Could you check a few things on this drawing? It's one solid part, dimensions in mm from its lowest x, y, z. A direction names the side the tool comes from. Give positions to 0.01 mm unless a question says otherwise; leave off trailing zeros. Order: outer loops, then holes, each group sorted by start corner. A loop starts at its lowest first (then second) coordinate and runs counter-clockwise, first axis right, second up.
(1) On a 3-axis mill with a long thin cutter (end or side, diameter ignored), from which of +Z, -Z, +X, -X, +Y, -Y can I reach the whole of each face in a straight line? I mean the marked faces 1, 2 and 3. Say none if no direction works.
(2) Imagine slicing it at A-A, the plane z = 12. State how many separate pieces and enclosed holes the cut face has.
(3) Imagine slicing it at B-B, the plane x = 14.5. Write out the boundary of the cut face in (y, z) (1 decimal).
(4) If I drill on probe 1 along Z at (x, y) = (8.5, 4.35) (1 decimal); probe 2 along X at (y, z) = (2.85, 18.5) (1 decimal); probe 3 along Z at (x, y) = (16, 4.05) (1 decimal), over which ranges is the centre line in solid material (lowest first)?
(5) Will these pins go through, and if not, where does the flat tip stop? pin 1 (1.5 mm diameter, centred on x = 18.5, y = 3.5, fed in from +Z); pin 2 (1.7 mm diameter, centred on x = 14.5, z = 5.39, fed in from -Y); pin 3 (3.5 mm diameter, centred on x = 12, z = 12, fed in from -Y); pin 4 (8 mm diameter, centred on x = 12, z = 12, fed in from +Y).
(6) If we mould it in two halves opening along Z, with no side actions, what happens to the marked faces 4, 5 and 6? For each: released by +Z, released by -Z, zero draft, split by the parting line, or undercut.
(7) Imagine slicing it at D-D, the plane y = 1.95. Write out the boundary of the cut face in (x, z).
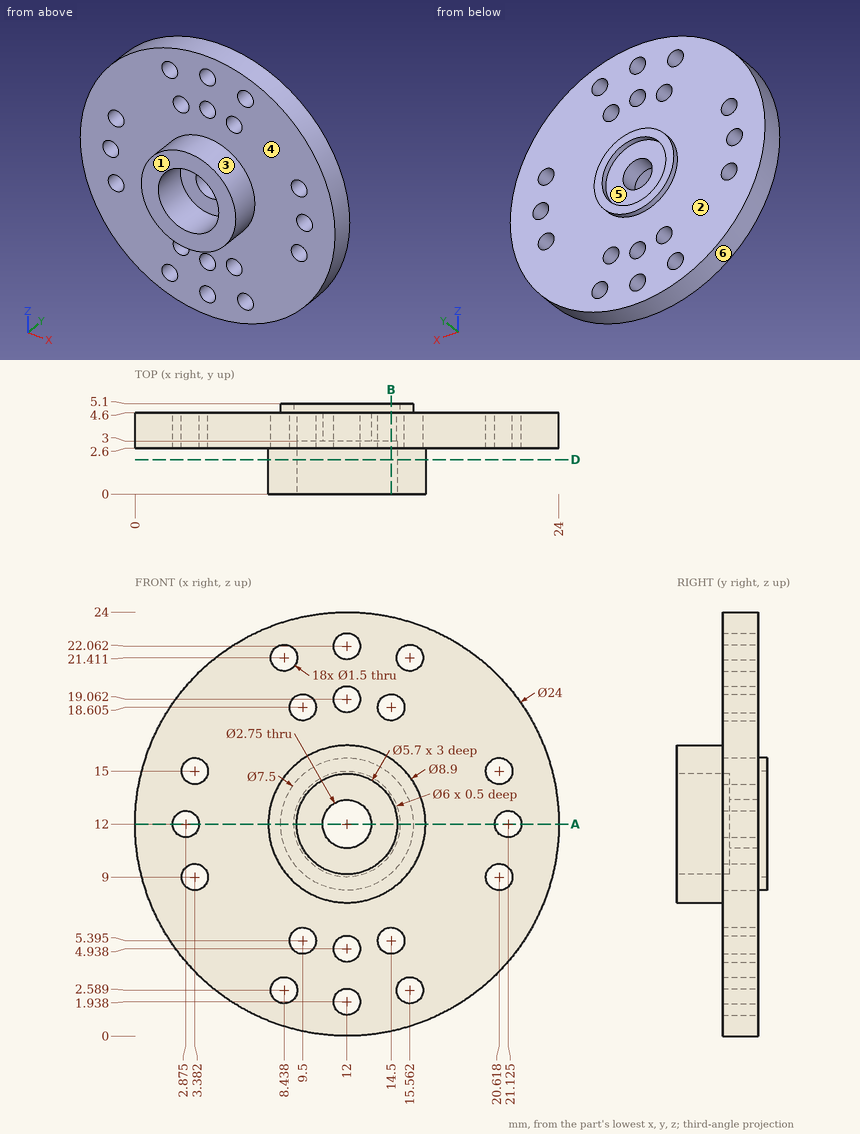
Answer block:
1. face 1: +Z, -Z, +X, -X, -Y
1. face 2: +Y
1. face 3: -Y
2. separate pieces: 4
2. enclosed holes: 0
3. outline: (0, 8.3) - (2.6, 8.3) - (2.6, 6.1) - (4.6, 6.1) - (4.6, 9.2) - (5.1, 9.2) - (5.1, 10.3) - (4.6, 10.3) - (4.6, 13.7) - (5.1, 13.7) - (5.1, 14.8) - (4.6, 14.8) - (4.6, 17.9) - (2.6, 17.9) - (2.6, 15.7) - (0, 15.7) - (0, 13.4) - (3, 13.4) - (3, 10.6) - (0, 10.6) - close; (2.6, 0.3) - (4.6, 0.3) - (4.6, 4.6) - (2.6, 4.6) - close; (2.6, 19.4) - (4.6, 19.4) - (4.6, 23.7) - (2.6, 23.7) - close
4. probe 1: z = 0.5 to 1.8, 3.3 to 20.7, 22.2 to 23.5
4. probe 2: x = 1.9 to 8.8, 10.2 to 11.5, 12.5 to 13.8, 15.2 to 22.1
4. probe 3: z = 0.7 to 2, 3.2 to 20.8, 22 to 23.3
5. pin 1: stops at z = 22.53
5. pin 2: stops at y = 2.6
5. pin 3: stops at y = 3
5. pin 4: stops at y = 5.1
6. face 4: zero draft
6. face 5: undercut
6. face 6: split by the parting line
7. outline: circle Ø8.9 at (12, 12); hole circle Ø5.7 at (12, 12)
